Geometry: see drawing. Coordinates: mm, zero at the bounding-box minimum. A direction names the side the tool comes from. Give positions to 0.01 mm unless a question says otherwise; leave off trailing zeros. Order: outer loops, then holes, each group sorted by start corner. A loop starts at its lowest first (then second) coordinate and runs counter-clockwise, first axis right, second up. Notation, with made-up numbers: M 42,-17.75 L 57,-17.75 A27 cw 57,11.25 Z; hole C -34,55.25 d1. An arc over 180 degrees is marked long. Return JSON: item names as keys, results as strings.
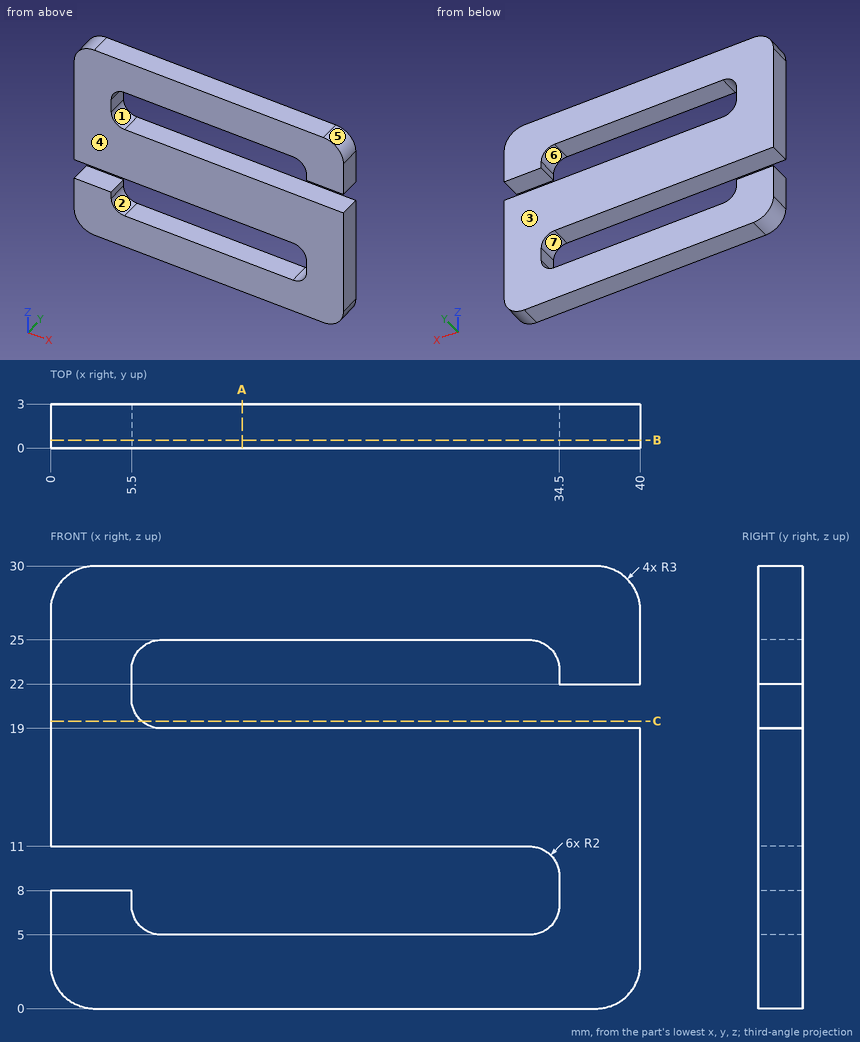
1. Ray query, probe 1 along Z at (x, y) = (11.5, 2.4); probe 2 along Z at (x, y) = (6, 1.7); probe 3 along X at (y, z) = (0.6, 8.5). Return the intervals inside material, ascending.
Evaluation:
{"probe 1": "z = 0 to 5, 11 to 19, 25 to 30", "probe 2": "z = 0 to 5.68, 11 to 19.68, 24.32 to 30", "probe 3": "x = 34.5 to 40"}
2. Draft query along X for the marked faces 4, 5, 6 and 7. Return one class per face: pulls with the +X half, pulls with the -X half, needs draft (parallel to the pull), parting line crosses it, or undercut.
Evaluation:
{"face 4": "needs draft", "face 5": "pulls with the +X half", "face 6": "undercut", "face 7": "pulls with the -X half"}
3. Section query B-B (y = 0.55). Return loops of the section in (x, z).
Evaluation:
{"outline": "M 0,3 A3 ccw 3,0 L 37,0 A3 ccw 40,3 L 40,19 L 7.5,19 A2 cw 5.5,21 L 5.5,23 A2 cw 7.5,25 L 32.5,25 A2 cw 34.5,23 L 34.5,22 L 40,22 L 40,27 A3 ccw 37,30 L 3,30 A3 ccw 0,27 L 0,11 L 32.5,11 A2 cw 34.5,9 L 34.5,7 A2 cw 32.5,5 L 7.5,5 A2 cw 5.5,7 L 5.5,8 L 0,8 Z"}
4. First-contact query: pin 1 (3 mm diameter, centred on x = 17, z = 24.5, fed in from -Y). Flat tip, straight axial feed; report the tip coordinate or a pass-through.
Evaluation:
{"pin 1": "stops at y = 0"}
5. Section query A-A (x = 13). Return loops of the section in (y, z), then the cut area to 3 significant figures.
Evaluation:
{"outline": "M 0,0 L 3,0 L 3,5 L 0,5 Z; M 0,11 L 3,11 L 3,19 L 0,19 Z; M 0,25 L 3,25 L 3,30 L 0,30 Z", "area": "54.0 mm^2"}
6. Section query C-C (z = 19.5). Return loops of the section in (x, y), then the cut area to 3 significant figures.
Evaluation:
{"outline": "M 0,0 L 6.18,0 L 6.18,3 L 0,3 Z", "area": "18.5 mm^2"}
7. Set-up query: the marked faces 1, 2 and 3. Return all of +Z, -Z, +X, -X, +Y, -Y with unobstructed straight access to the full face (end or side cutting, diameter ignored); none if empty.
Evaluation:
{"face 1": "+X, +Y, -Y", "face 2": "+Y, -Y", "face 3": "+Z, -Z, +X, -X, +Y"}
